Geometry check sheet. Reference: the model listing, model coordinates, mm. Face numbers are marked on the shaded views. Give positions to 0.01 mm unless a question says otherwise; leave off trailing zeros. Write each loop counter-clockwise with the first axis right and the second up, starting at its lowest first coordinate (ties: lowest second). Pieces come first, ordered by that corner, then holes. Notation, with made-up numbers: (40.5, 60.25) - (99.5, 60.25) arc R7 cw to (99.5, 69.25) - close; hole circle Ø5 at (-31, 19.25). An arc over 180 degrees is marked (long way). Write item = value, one per line. Start each with the question number.
(1) Section check B-B, the plane y = -129.5. Enter the section's corners in (x, z), plus the area to 3 significant figures.
(2) Section check C-C, the plane x = -16.5. Enter the section's corners in (y, z).
(3) Thickness scan on L1, parallel to X at y = -37.78, z = 0.5; L2, parallel to X at y = -32.7, z = 0.85; L3, parallel to Y at x = 12.5, z = -27. Record the ranges inside material, lowest first.
(4) Section check A-A, the plane z = -10.5. Enter the section's corners in (x, y), plus the area to 3 significant figures.
(5) Draft check along X on the marked faces 1 and 2. Enter one of: pulls with the +X half, pulls with the -X half, needs draft (parallel to the pull), parting line crosses it, or undercut.
(6) Section check D-D, the plane x = 15.5. Enter the section's corners in (y, z), plus the area to 3 significant figures.
(7) Depth check by flat-ended pin: pin 1 Ø3 at (y, z) = (-130, -2) entering from -X; pin 2 Ø12 at (x, z) = (12, -15.5) entering from +Y; pin 3 Ø5 at (x, y) = (-19, -39) entering from -Z. Enter the tip coordinate at first touch or a pass-through.
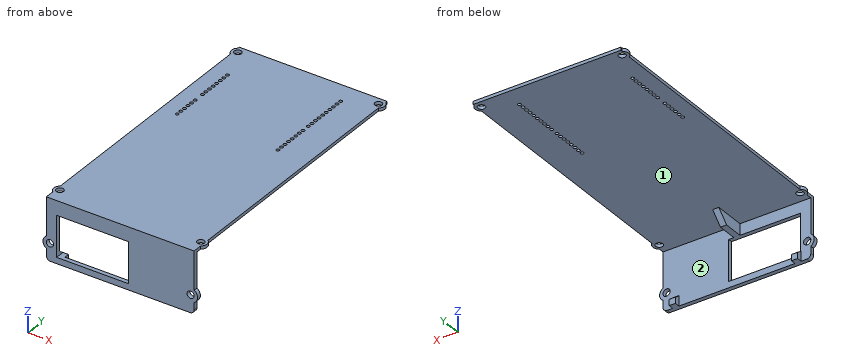
```python
from build123d import *

# Parameters (mm, degrees)
SKETCH1_R                = 1.75
BOSS_EXTRUDE1_DEPTH      = 1.5
BOSS_EXTRUDE2_DEPTH      = 72
BOSS_EXTRUDE3_DEPTH      = 1.5
BOSS_EXTRUDE3_DEPTH_BACK = 1.5
BOSS_EXTRUDE4_DEPTH      = 2
SKETCH5_R                = 1.75
CUT_EXTRUDE1_DEPTH       = 2
CUT_EXTRUDE2_DEPTH       = 148.332054879
CUT_EXTRUDE2_DEPTH_BACK  = 148.332054879
SKETCH6_W                = 72
SKETCH6_H                = 11.553195909
BOSS_EXTRUDE6_START      = -2
SKETCH7_W                = 3
SKETCH7_H                = 4
BOSS_EXTRUDE6_DEPTH      = 2.5
FILLET1_R                = 2
CHAMFER1_SIZE            = 1
FILLET2_R                = 8
SKETCH8_W                = 35
SKETCH8_H                = 19.946804091
CUT_EXTRUDE3_DEPTH       = 22.4262221
SKETCH10_R               = 0.8
CUT_EXTRUDE4_DEPTH       = 1.5


with BuildPart() as part:
    # Sketch1 → Boss-Extrude1 (new body)
    with BuildSketch(Plane.XY):
        with BuildLine():
            Line((-31.5, -134.5), (31.5, -134.5))
            Line((31.5, -134.5), (36, -134.5))
            Line((36, -134.5), (36, -132.049019419))
            ThreePointArc((36, -132.049019419), (37.374296294, -129.5), (36, -126.950980581))
            Line((36, -126.950980581), (36, -6.049019419))
            ThreePointArc((36, -6.049019419), (37.33874188, -3.5), (36, -0.950980581))
            Line((36, -0.950980581), (36, 0))
            Line((36, 0), (-36, 0))
            Line((-36, 0), (-36, -0.950980581))
            ThreePointArc((-36, -0.950980581), (-37.339851511, -3.504206195), (-35.994020506, -6.054285021))
            Line((-35.994020506, -6.054285021), (-36, -126.950980581))
            ThreePointArc((-36, -126.950980581), (-37.376731289, -129.5), (-36, -132.049019419))
            Line((-36, -132.049019419), (-36, -134.5))
            Line((-36, -134.5), (-31.5, -134.5))
        make_face()
        with Locations((-34.328609587, -129.5)):
            Circle(SKETCH1_R, mode=Mode.SUBTRACT)
        with Locations((34.323211043, -129.5)):
            Circle(SKETCH1_R, mode=Mode.SUBTRACT)
        with Locations((34.242652207, -3.5)):
            Circle(SKETCH1_R, mode=Mode.SUBTRACT)
        with Locations((-34.244120111, -3.500578956)):
            Circle(SKETCH1_R, mode=Mode.SUBTRACT)
    extrude(amount=BOSS_EXTRUDE1_DEPTH)

    # Sketch2 → Boss-Extrude2 (add)
    with BuildSketch(Plane.ZY.offset(36)):
        Polygon((1.5, -134.5), (1.5, -136.7), (-40, -136.7), (-40, -134.7), (0, -134.7), (0, -134.5), (0, -132.049019419), (1.5, -132.049019419), align=None)
    extrude(amount=-BOSS_EXTRUDE2_DEPTH)

    # Sketch3 → Boss-Extrude3 (add, two sides: drawn at the far end of the back side and taken through both)
    with BuildSketch(Plane(origin=(0, 0, 0), x_dir=(0, 0, -1), z_dir=(1, 0, 0)).offset(-BOSS_EXTRUDE3_DEPTH_BACK)):
        Polygon((0, -119.7), (15, -134.7), (0, -134.7), align=None)
    extrude(amount=BOSS_EXTRUDE3_DEPTH + BOSS_EXTRUDE3_DEPTH_BACK)

    # Sketch4 → Boss-Extrude4 (add)
    with BuildSketch(Plane.XZ.offset(136.7)):
        with BuildLine():
            Line((-36, -17.152805247), (-36, -22.963011674))
            ThreePointArc((-36, -22.963011674), (-37.650416645, -20.05790846), (-36, -17.152805247))
        make_face()
        with BuildLine():
            Line((36, -17.152805247), (36, -22.963011674))
            ThreePointArc((36, -22.963011674), (37.68082264, -20.05790846), (36, -17.152805247))
        make_face()
    extrude(amount=-BOSS_EXTRUDE4_DEPTH)

    # Sketch5 → Cut-Extrude1 (cut)
    with BuildSketch(Plane.XZ.offset(136.7)):
        with Locations(Location((-34.253947115, -19.946804091, 0), (0, 0, 270))):
            Circle(SKETCH5_R)
        with Locations(Location((34.288977705, -19.889159472, 0), (0, 0, 270))):
            Circle(SKETCH5_R)
    extrude(amount=-CUT_EXTRUDE1_DEPTH, mode=Mode.SUBTRACT)

    # Sketch6 → Cut-Extrude2 (cut, two sides: drawn at the far end of the back side and taken through both)
    with BuildSketch(Plane.XZ.offset(136.7).offset(-CUT_EXTRUDE2_DEPTH_BACK)):
        with Locations((0, -34.223402046)):
            Rectangle(SKETCH6_W, SKETCH6_H)
    extrude(amount=CUT_EXTRUDE2_DEPTH + CUT_EXTRUDE2_DEPTH_BACK, mode=Mode.SUBTRACT)

    # Sketch7 → Boss-Extrude6 (add)
    with BuildSketch(Plane.XZ.offset(136.7).offset(BOSS_EXTRUDE6_START)):
        with Locations((-29.8, -26.446804091)):
            Rectangle(SKETCH7_W, SKETCH7_H)
        with Locations((29.8, -26.446804091)):
            Rectangle(SKETCH7_W, SKETCH7_H)
    extrude(amount=-BOSS_EXTRUDE6_DEPTH)

    # Fillet1
    fillet1_edges = [part.edges().sort_by_distance(p)[0] for p in [
        (36, -135.7, -28.446804091),
        (-36, -135.7, -28.446804091),
    ]]
    fillet(fillet1_edges, radius=FILLET1_R)

    # Chamfer1
    chamfer1_edges = [part.edges().sort_by_distance(p)[0] for p in [
        (-29.8, -134.7, -24.446804091),
        (-29.8, -132.2, -24.446804091),
        (29.8, -134.7, -24.446804091),
        (29.8, -132.2, -24.446804091),
    ]]
    chamfer(chamfer1_edges, length=CHAMFER1_SIZE)

    # Fillet2
    # the kernel refuses this fillet: 8 mm, written as the material it takes off along each edge
    with BuildSketch(Plane(origin=(-23.303909917, -133.2, -24.446804091), x_dir=(0, -1.0, -1.118394266079786e-11), z_dir=(-1, 0, 0))) as fillet2_piece_1:
        with BuildLine():
            CenterArc((4.243746579, -7.06996192), FILLET2_R, 117.902496562, 17.097503438)
            Line((-1.413107671, -1.413107671), (0, 0))
            Line((0, 0), (0.5, 0))
        make_face()
    extrude(amount=12.992180166, mode=Mode.SUBTRACT)
    with BuildSketch(Plane(origin=(23.303909917, -133.2, -24.446804091), x_dir=(0, 0.7071067811865476, -0.7071067811865476), z_dir=(1, 0, 0))) as fillet2_piece_2:
        with BuildLine():
            CenterArc((1.998436033, -8), FILLET2_R, 90, 17.097503438)
            Line((-0.353553391, -0.353553391), (0, 0))
            Line((0, 0), (1.998436033, 0))
        make_face()
    extrude(amount=12.992180166, mode=Mode.SUBTRACT)

    # Sketch8 → Cut-Extrude3 (cut)
    with BuildSketch(Plane.XZ.offset(136.7)):
        with Locations((-13.5, -15.473402046)):
            Rectangle(SKETCH8_W, SKETCH8_H)
    extrude(amount=-CUT_EXTRUDE3_DEPTH, mode=Mode.SUBTRACT)

    # Sketch10 → Cut-Extrude4 (cut)
    with BuildSketch(Plane.XY.offset(1.5)):
        with Locations((-27.994710245, -20)):
            Circle(SKETCH10_R)
        with Locations((-27.994710245, -22.54)):
            Circle(SKETCH10_R)
        with Locations((-27.994710245, -25.08)):
            Circle(SKETCH10_R)
        with Locations((-27.994710245, -27.62)):
            Circle(SKETCH10_R)
        with Locations((-27.994710245, -30.16)):
            Circle(SKETCH10_R)
        with Locations((-27.994710245, -32.7)):
            Circle(SKETCH10_R)
        with Locations((-27.994710245, -35.24)):
            Circle(SKETCH10_R)
        with Locations((-27.994710245, -37.78)):
            Circle(SKETCH10_R)
        with Locations((20.605289755, -10.5)):
            Circle(SKETCH10_R)
        with Locations((-27.994710245, -42.86)):
            Circle(SKETCH10_R)
        with Locations((-27.994710245, -45.4)):
            Circle(SKETCH10_R)
        with Locations((-27.994710245, -47.94)):
            Circle(SKETCH10_R)
        with Locations((-27.994710245, -50.48)):
            Circle(SKETCH10_R)
        with Locations((-27.994710245, -53.02)):
            Circle(SKETCH10_R)
        with Locations((-27.994710245, -55.56)):
            Circle(SKETCH10_R)
        with Locations((20.605289755, -13.04)):
            Circle(SKETCH10_R)
        with Locations((20.605289755, -15.58)):
            Circle(SKETCH10_R)
        with Locations((20.605289755, -18.12)):
            Circle(SKETCH10_R)
        with Locations((20.605289755, -20.66)):
            Circle(SKETCH10_R)
        with Locations((20.605289755, -23.2)):
            Circle(SKETCH10_R)
        with Locations((20.605289755, -25.74)):
            Circle(SKETCH10_R)
        with Locations((20.605289755, -28.28)):
            Circle(SKETCH10_R)
        with Locations((20.605289755, -30.82)):
            Circle(SKETCH10_R)
        with Locations((20.605289755, -33.36)):
            Circle(SKETCH10_R)
        with Locations((20.605289755, -37.16)):
            Circle(SKETCH10_R)
        with Locations((20.605289755, -39.7)):
            Circle(SKETCH10_R)
        with Locations((20.605289755, -42.24)):
            Circle(SKETCH10_R)
        with Locations((20.605289755, -44.78)):
            Circle(SKETCH10_R)
        with Locations((20.605289755, -47.32)):
            Circle(SKETCH10_R)
        with Locations((20.605289755, -49.86)):
            Circle(SKETCH10_R)
        with Locations((20.605289755, -52.4)):
            Circle(SKETCH10_R)
        with Locations((20.605289755, -54.94)):
            Circle(SKETCH10_R)
    extrude(amount=-CUT_EXTRUDE4_DEPTH, mode=Mode.SUBTRACT)


solid = part.part
```
Model answer:
q1.outline = (-37.38, 0) - (-36.08, 0) - (-36.08, 1.5) - (-37.38, 1.5) - close; (-32.58, 0) - (-1.5, 0) - (-1.5, -5.5) - (1.5, -5.5) - (1.5, 0) - (32.57, 0) - (32.57, 1.5) - (-32.58, 1.5) - close; (36.07, 0) - (37.37, 0) - (37.37, 1.5) - (36.07, 1.5) - close
q1.area = 118 mm²
q2.outline = (-136.7, -28.45) - (-134.7, -28.45) - (-134.7, -25.45) - (-136.7, -25.45) - close; (-136.7, -5.5) - (-134.7, -5.5) - (-134.7, 0) - (0, 0) - (0, 1.5) - (-136.7, 1.5) - close
q3.L1 = -36 to -28.79, -27.19 to 20.1, 21.11 to 36
q3.L2 = -36 to -28.79, -27.19 to 20.15, 21.06 to 36
q3.L3 = -136.7 to -134.7
q4.outline = (-36, -136.7) - (-31, -136.7) - (-31, -134.7) - (-36, -134.7) - close; (4, -136.7) - (36, -136.7) - (36, -134.7) - (4, -134.7) - close
q4.area = 74.0 mm²
q5.face_1 = needs draft
q5.face_2 = undercut
q6.outline = (-136.7, -28.45) - (-134.7, -28.45) - (-134.7, 0) - (0, 0) - (0, 1.5) - (-136.7, 1.5) - close
q6.area = 262 mm²
q7.pin_1 = -1.5
q7.pin_2 = -134.7
q7.pin_3 = 0
